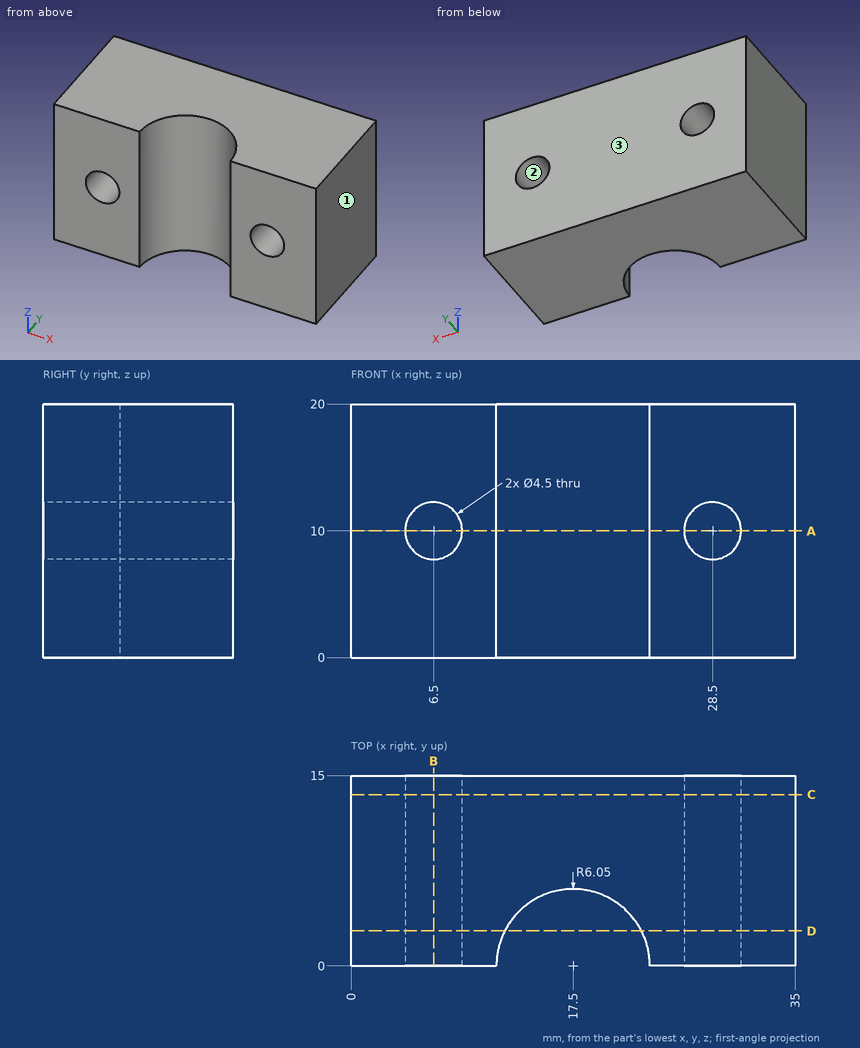
Could you check a few things on this drawing? It's one solid part, dimensions in mm from its lowest x, y, z. Round coordinates to 2 decimals unless told otherwise and drop trailing zeros. Write each loop counter-clockwise with the first axis right and the second up, starting at its lowest first coordinate (ties: lowest second). Pieces come first, ordered by that corner, then holes. Notation, with made-up numbers: (69, 2) -> (114, 2) arc R20 ccw to (114, 27) -> close; hole circle Ø1 at (-32.75, 58.5). An arc over 180 degrees is marked (long way). One line per question, with ' | ' between items. Start each with the question number.
1) Suppose I cut it at B-B on x = 6.5. Write out the boundary of the cut face in (y, z).
2) I'm going to push a flat-ended pin straight in: P1, Ø3.5, axis at x = 6.5, z = 10, coming from the -Y side. Where does the tip first touch, or does it pass through?
3) I need wall thicknesses on line 1 (Z direction, x = 6.5, y = 12.5); line 2 (X direction, y = 4, z = 15.5); line 3 (X direction, y = 4.25, z = 3.75). Which ranges of each line are inside material? Lowest first, please. Write a range as [from, to].
4) Suppose I cut it at C-C on y = 13.5. Write out the boundary of the cut face in (x, z), then the cut area to 3 significant figures.
5) Suppose I cut it at D-D on y = 2.75. Write out the boundary of the cut face in (x, z).
6) If we mould it in two halves opening along X, with no side actions, what happens to the marked faces 1, 2 and 3? For each: released by +X, released by -X, zero draft, split by the parting line, or undercut.
7) Suppose I cut it at A-A on z = 10. Write out the boundary of the cut face in (x, y), then the cut area to 3 significant figures.
Return value:
1) outline: (0, 0) -> (15, 0) -> (15, 7.75) -> (0, 7.75) -> close; (0, 12.25) -> (15, 12.25) -> (15, 20) -> (0, 20) -> close
2) P1: passes through
3) line 1: z = [0, 7.75], [12.25, 20] | line 2: x = [0, 12.96], [22.04, 35] | line 3: x = [0, 13.19], [21.81, 35]
4) outline: (0, 0) -> (35, 0) -> (35, 20) -> (0, 20) -> close; hole circle Ø4.5 at (6.5, 10); hole circle Ø4.5 at (28.5, 10) | area: 668 mm2
5) outline: (0, 0) -> (12.11, 0) -> (12.11, 20) -> (0, 20) -> close; (22.89, 0) -> (35, 0) -> (35, 20) -> (22.89, 20) -> close; hole circle Ø4.5 at (6.5, 10); hole circle Ø4.5 at (28.5, 10)
6) face 1: released by +X | face 2: undercut | face 3: zero draft
7) outline: (0, 0) -> (4.25, 0) -> (4.25, 15) -> (0, 15) -> close; (8.75, 0) -> (11.45, 0) arc R6.05 cw to (23.55, 0) -> (26.25, 0) -> (26.25, 15) -> (8.75, 15) -> close; (30.75, 0) -> (35, 0) -> (35, 15) -> (30.75, 15) -> close | area: 333 mm2
